Read the model definition and answer for the solid it produces. Units are mm, in the model's axes. Coordinates: 2 decimals unless noted, no trailing zeros. Order: outer loops, then holes, each group sorted by start corner. A loop starts at its lowest first (then second) coordinate and runs counter-clockwise, first axis right, second up. Notation, with made-up numbers: (34, 38) -> (84, 38) arc R17 cw to (84, 43) -> close; hole circle Ø11 at (46.5, -7.75). An arc over 180 degrees is marked (long way). Answer in a Markdown table with one row per item.
from build123d import *

# Parameters (mm, degrees)
BOSS_EXTRUDE2_DEPTH      = 5
BOSS_EXTRUDE2_DEPTH_BACK = 10
SKETCH1_W                = 120.517011816
SKETCH1_H                = 193.423301164
CUT_EXTRUDE1_DEPTH       = 117.520998071
CUT_EXTRUDE1_DEPTH_BACK  = 117.520998071
SKETCH2_W                = 10.720124134
SKETCH2_H                = 2
SKETCH2_W_2              = 57.651632978
SKETCH2_W_3              = 14.145254704
CUT_EXTRUDE2_START       = -95.651632978
CUT_EXTRUDE2_DEPTH       = 95.651632978
CUT_EXTRUDE4_DEPTH       = 156.859658163
CUT_EXTRUDE4_DEPTH_BACK  = 156.859658163
SKETCH5_W                = 11
SKETCH5_H                = 191.423301164
BOSS_EXTRUDE3_DEPTH      = 10
BOSS_EXTRUDE3_DRAFT      = 70
BOSS_EXTRUDE4_DEPTH      = 5
BOSS_EXTRUDE4_TAPER      = 17


# Read off the part's stored shape, not the designer's step: Cut-Extrude2
with BuildPart() as part:
    # Sketch1 → Boss-Extrude2 (new, two sides: drawn at the far end of the back side and taken through both)
    with BuildSketch(Plane.XY.offset(-BOSS_EXTRUDE2_DEPTH_BACK)):
        with Locations((0.408269184, 1.633076737)):
            Rectangle(SKETCH1_W, SKETCH1_H)
    extrude(amount=BOSS_EXTRUDE2_DEPTH + BOSS_EXTRUDE2_DEPTH_BACK)

    # Sketch2 → Cut-Extrude1 (cut, two sides: drawn at the far end of the back side and taken through both)
    with BuildSketch(Plane(origin=(0, 0, -10), x_dir=(-1, 0, 0), z_dir=(0, 0, -1)).offset(-CUT_EXTRUDE1_DEPTH_BACK)):
        with Locations((-55.306713025, 97.344727319)):
            Rectangle(SKETCH2_W, SKETCH2_H)
        with Locations((-2.120834469, 97.344727319)):
            Rectangle(SKETCH2_W_2, SKETCH2_H)
        with Locations((52.777609372, 97.344727319)):
            Rectangle(SKETCH2_W_3, SKETCH2_H)
    extrude(amount=CUT_EXTRUDE1_DEPTH + CUT_EXTRUDE1_DEPTH_BACK, mode=Mode.SUBTRACT)

    # Cut-Extrude2 outline → Cut-Extrude2 (cut)
    with BuildSketch(Plane(origin=(49.946650958, 0, 0), x_dir=(0, 0, -1), z_dir=(1, 0, 0)).offset(CUT_EXTRUDE2_START)):
        with BuildLine():
            Line((-5, 96.344727319), (8.880031812, 96.344727322))
            add(Edge.make_bspline(
                [(8.880031812, 96.344727322), (9.017757925, 96.389418818), (9.341148133, 96.502947325), (9.65511797, 96.721266154), (9.834207861, 97.091812499), (9.772304841, 97.682742311), (9.591846004, 97.952667933), (9.299739635, 98.085555426), (8.979382301, 98.13209035), (8.595809552, 98.122046866), (8.280683269, 98.057581679), (8.068335475, 97.930949515), (7.924267823, 97.772346881), (7.828035074, 97.54375556), (7.790578102, 97.292694013), (7.792508646, 97.124503178), (7.79875666, 97.046103501)],
                knots=[0.210157703, 0.210157703, 0.210157703, 0.210157703, 0.25, 0.3125, 0.375, 0.5, 0.625, 0.6875, 0.75, 0.8125, 0.875, 0.90625, 0.9375, 0.96875, 0.984375, 1, 1, 1, 1], degree=3))
            Line((7.79875666, 97.046103501), (7.599388771, 97.030214998))
            add(Edge.make_bspline(
                [(10, 97.255513039), (9.999998961, 97.447527895), (9.972419046, 97.629851143), (9.927722494, 97.794553197), (9.870710413, 97.937325839), (9.798783484, 98.058137149), (9.704435395, 98.159491912), (9.580897677, 98.243174202), (9.426924325, 98.307669655), (9.246866395, 98.348516931), (9.047009529, 98.36212633), (8.833423752, 98.351560976), (8.612813999, 98.330782958), (8.391619774, 98.318858897), (8.17208277, 98.31353746), (7.941741695, 98.247701653), (7.690138593, 98.003146143), (7.552784018, 97.615008356), (7.599388771, 97.030214998)],
                knots=[0.42378525, 0.42378525, 0.42378525, 0.42378525, 0.42378525, 0.42378525, 0.42378525, 0.42378525, 0.42378525, 0.42378525, 0.42378525, 0.42378525, 0.42378525, 0.42378525, 0.42378525, 0.42378525, 0.42378525, 0.42378525, 0.42378525, 1, 1, 1, 1, 1, 1, 1, 1, 1, 1, 1, 1, 1, 1, 1, 1, 1, 1, 1], degree=18))
            Line((10, 97.255513039), (10, 98.344727319))
            Line((10, 98.344727319), (-5, 98.344727319))
            Line((-5, 98.344727319), (-5, 96.344727319))
        make_face()
    extrude(amount=CUT_EXTRUDE2_DEPTH, mode=Mode.SUBTRACT)

    # Sketch5 → Cut-Extrude4 (cut, two sides: drawn at the far end of the back side and taken through both)
    with BuildSketch(Plane(origin=(60.666775092, 0, 0), x_dir=(0, 0, -1), z_dir=(1, 0, 0)).offset(-CUT_EXTRUDE4_DEPTH_BACK)):
        with Locations((0.5, 0.633076737)):
            Rectangle(SKETCH5_W, SKETCH5_H)
    extrude(amount=CUT_EXTRUDE4_DEPTH + CUT_EXTRUDE4_DEPTH_BACK, mode=Mode.SUBTRACT)


with BuildPart() as boss_extrude3_tool:
    # Sketch6 → Boss-Extrude3 (with draft: the straight prism first)
    with BuildSketch(Plane(origin=(0, 0, -10), x_dir=(-1, 0, 0), z_dir=(0, 0, -1))):
        Polygon((-49.946650958, 96.344727319), (-60.666775092, 96.344727319), (-60.666775092, -95.078573845), (59.850236724, -95.078573845), (59.850236724, 96.344727319), (45.70498202, 96.344727319), (26.70498202, 96.344727319), (-30.946650958, 96.344727319), align=None)
    extrude(amount=BOSS_EXTRUDE3_DEPTH)
    # Boss-Extrude3: the draft: its side faces are tilted about the plane it starts from
    boss_extrude3_sides = [boss_extrude3_tool.faces().sort_by_distance(p)[0] for p in [
        (0.408269184, 96.344727319, -15),
        (60.666775092, 0.633076737, -15),
        (0.408269184, -95.078573845, -15),
        (-59.850236724, 0.633076737, -15),
    ]]
    draft(boss_extrude3_sides, Plane(origin=(0, 0, -10), x_dir=(-1, 0, 0), z_dir=(0, 0, -1)), BOSS_EXTRUDE3_DRAFT)


with BuildPart() as part_1:
    add(part.part)

    # Boss-Extrude3: add boss_extrude3_tool
    add(boss_extrude3_tool.part)

    # Sketch7 → Boss-Extrude4 (add)
    with BuildSketch(Plane(origin=(0, 0, -20), x_dir=(-1, 0, 0), z_dir=(0, 0, -1))):
        with BuildLine():
            ThreePointArc((-11.292084394, -51.674806102), (-0.79402055, -59.989504928), (9.681667321, -51.646632242))
            ThreePointArc((9.681667321, -51.646632242), (8.230968391, -49.324207989), (5.908544137, -50.774906919))
            ThreePointArc((5.908544137, -50.774906919), (-0.79922246, -56.116994562), (-7.521316785, -50.792947135))
            ThreePointArc((-7.521316785, -50.792947135), (-9.847630073, -49.348492814), (-11.292084394, -51.674806102))
        make_face()
    extrude(amount=BOSS_EXTRUDE4_DEPTH, taper=BOSS_EXTRUDE4_TAPER)


solid = part_1.part
Q1. The part is cut by section B-B (x = -48.5). Write down the section's boundary in (y, z), then the cut area to 3 significant figures.
Outcome:
| item | result |
|---|---|
| outline | (-95.08, -10) -> (-83.73, -14.13) -> (84.99, -14.13) -> (96.34, -10) -> (96.34, -6) -> (-95.08, -6) -> close |
| area | 1,510 mm² |
Q2. Given pin 1 (1.2 mm diameter, centred on x = -55, z = -8, fed in from +Y); pin 2 (6 mm diameter, centred on x = 20.5, z = -11, fed in from -Y); pin 3 (4 mm diameter, centred on x = -13.5, y = -33, fed in from -Z); pin 4 (1.6 mm diameter, centred on y = 98, z = -8, fed in from +X), each flat-ended and moving along its own axis, determine where each tip first touches the part or whether it passes through.
Outcome:
| item | result |
|---|---|
| pin 1 | y = 96.34 |
| pin 2 | y = -95.08 |
| pin 3 | z = -20 |
| pin 4 | x = 49.95 |
Q3. Consider line 1 (Z direction, x = 19, y = -21.5); line 2 (Y direction, x = 33, z = -8); line 3 (Y direction, x = 30, z = -9.75). Determine where each line is inside the solid, lowest interval first.
Outcome:
| item | result |
|---|---|
| line 1 | -20 to -6 |
| line 2 | -95.08 to 96.34, 97.85 to 98.12 |
| line 3 | -95.08 to 96.34 |
Q4. The part is cut by section A-A (y = -41). Write down the section's boundary in (x, z), then the cut area to 3 significant figures.
Outcome:
| item | result |
|---|---|
| outline | (-59.85, -10) -> (-32.38, -20) -> (33.19, -20) -> (60.67, -10) -> (60.67, -6) -> (-59.85, -6) -> close |
| area | 1,410 mm² |
Q5. The part is cut by section C-C (z = -17). Write down the section's boundary in (x, y).
Outcome:
| item | result |
|---|---|
| outline | (-40.62, -75.85) -> (41.43, -75.85) -> (41.43, 77.11) -> (-40.62, 77.11) -> close |
